The model under review builds one solid part; all positions refer to its coordinate system, in mm. A direction names the side the tool comes from. Coordinates: 2 decimals unless noted, no trailing zeros. Order: outer loops, then holes, each group sorted by start corner. A loop starts at its lowest first (then second) coordinate and runs counter-clockwise, first axis right, second up. Notation, with made-up numbers: (73.25, 49) -> (107.25, 49) arc R23 cw to (107.25, 83) -> close; hole circle Ø2 at (55.5, 88.25). An arc over 180 degrees is marked (long way). Use one line per item in the form item = value. Start each with the question number.
(1) Take a section at B-B (x = -4.5). State the section outline as (y, z) points, then the cut area to 3 significant figures.
(2) Take a section at A-A (y = -46). State the section outline as (x, z) points, then the cut area to 3 significant figures.
(3) Take a section at D-D (y = -24.5). State the section outline as (x, z) points.
(4) Insertion check: pin 1 Ø5.5 at (x, z) = (-18, 1.5) entering from -Y; pin 2 Ø1.5 at (x, y) = (-9.5, -18.5) entering from -Z; pin 3 Ø12 at (x, z) = (-1.5, 22) entering from +Y; pin 4 Ø21 at (x, y) = (-2.5, 5.5) entering from +Z. Each pin has a flat end and moves straight along its axis. Give the tip position at first contact, or say it passes through.
(5) For faces 5 (the flat face through (17, -35.5, 2)), 6 (the flat face through (-25.6, 27, 5)), 7 (the cylindrical face through (-6.232, -28.066, 6.479)), list the 3-axis set-ups (+Z, -Z, +X, -X, +Y, -Y) from which the entire face can be reached by the end or side of a thin tool; tool diameter is ignored.
(6) Take a section at C-C (z = 19.5). State the section outline as (x, y) points.
(7) Mouldability with a two-part tool opening along X and no side actions: class faces 1 (the cylindrical face through (29.038, 26.004, 2.465)), 2 (the cylindrical face through (33.245, -33.361, 2.465)), 3 (the flat face through (27, 25.7, 5)), 4 (the cylindrical face through (-33.361, -33.245, 2.465)) as +X half, -X half, draft (parallel to the pull), parting line (faces both ways), or undercut.
(8) Wall thickness on line 1 along Y through (x, z) = (28, 3.7); line 2 along Y through (x, z) = (0, 9.7); line 3 along Z through (x, y) = (-19.5, 16): over which ranges is each line inside the solid? List them lowest first.
```python
from build123d import *

# Parameters (mm, degrees)
SKETCH004_R         = 2.25
SKETCH004_R_2       = 11.1
SKETCH004_R_3       = 1.65
PAD005_DEPTH        = 5
SKETCH005_R         = 35.5
SKETCH005_R_2       = 32.6
PAD006_DEPTH        = 8
SKETCH070_R         = 32.6
SKETCH070_R_2       = 28.75
PAD045_DEPTH        = 3
SKETCH071_W         = 11
SKETCH071_H         = 18
SKETCH071_R         = 1.0922
PAD046_DEPTH        = 25.5
HOLE002_D           = 3.4
HOLE002_CSINK_D     = 6.7
HOLE002_CSINK_ANGLE = 90


with BuildPart() as part:
    # Sketch004 → Pad005 (new body)
    with BuildSketch(Plane.XY):
        with BuildLine():
            Line((-28, 35.5), (28, 35.5))
            ThreePointArc((35.5, 28), (33.303301, 33.303301), (28, 35.5))
            Line((35.5, 28), (35.5, -28))
            ThreePointArc((28, -35.5), (33.303301, -33.303301), (35.5, -28))
            Line((28, -35.5), (-28, -35.5))
            ThreePointArc((-35.5, -28), (-33.303301, -33.303301), (-28, -35.5))
            Line((-35.5, -28), (-35.5, 28))
            ThreePointArc((-28, 35.5), (-33.303301, 33.303301), (-35.5, 28))
        make_face()
        with Locations((-28, 28)):
            Circle(SKETCH004_R, mode=Mode.SUBTRACT)
        with Locations((28, 28)):
            Circle(SKETCH004_R, mode=Mode.SUBTRACT)
        with Locations((28, -28)):
            Circle(SKETCH004_R, mode=Mode.SUBTRACT)
        with Locations((-28, -28)):
            Circle(SKETCH004_R, mode=Mode.SUBTRACT)
        Circle(SKETCH004_R_2, mode=Mode.SUBTRACT)
        with Locations((-9.899495, 9.899495)):
            Circle(SKETCH004_R_3, mode=Mode.SUBTRACT)
        with Locations((9.899495, 9.899495)):
            Circle(SKETCH004_R_3, mode=Mode.SUBTRACT)
        with Locations((9.899495, -9.899495)):
            Circle(SKETCH004_R_3, mode=Mode.SUBTRACT)
        with Locations((-9.899495, -9.899495)):
            Circle(SKETCH004_R_3, mode=Mode.SUBTRACT)
    extrude(amount=PAD005_DEPTH)

    # Sketch005 → Pad006 (join)
    with BuildSketch(Plane.XY.offset(5)):
        Circle(SKETCH005_R)
        Circle(SKETCH005_R_2, mode=Mode.SUBTRACT)
    extrude(amount=PAD006_DEPTH)

    # Sketch070 → Pad045 (join)
    with BuildSketch(Plane.XY.offset(5)):
        Circle(SKETCH070_R)
        Circle(SKETCH070_R_2, mode=Mode.SUBTRACT)
    extrude(amount=PAD045_DEPTH)

    # Sketch071 → Pad046 (join)
    with BuildSketch(Plane.XY):
        with Locations((-0.5, -42)):
            Rectangle(SKETCH071_W, SKETCH071_H)
        with Locations((0, -38)):
            Circle(SKETCH071_R, mode=Mode.SUBTRACT)
        with Locations((0, -46)):
            Circle(SKETCH071_R, mode=Mode.SUBTRACT)
    extrude(amount=PAD046_DEPTH)

    # Hole002 (through all)
    with Locations(Plane.XY.offset(5)):
        with Locations((-9.899495, 9.899495), (9.899495, 9.899495), (9.899495, -9.899495), (-9.899495, -9.899495)):
            CounterSinkHole(HOLE002_D / 2, HOLE002_CSINK_D / 2, counter_sink_angle=HOLE002_CSINK_ANGLE)


solid = part.part
```
Findings:
q1.outline = (-51, 0) -> (-10.15, 0) -> (-10.15, 5) -> (-28.4, 5) -> (-28.4, 8) -> (-32.29, 8) -> (-32.29, 13) -> (-33, 13) -> (-33, 25.5) -> (-51, 25.5) -> close; (10.15, 0) -> (35.5, 0) -> (35.5, 5) -> (35.21, 5) -> (35.21, 13) -> (32.29, 13) -> (32.29, 8) -> (28.4, 8) -> (28.4, 5) -> (10.15, 5) -> close
q1.area = 752 mm²
q2.outline = (-6, 0) -> (-1.09, 0) -> (-1.09, 25.5) -> (-6, 25.5) -> close; (1.09, 0) -> (5, 0) -> (5, 25.5) -> (1.09, 25.5) -> close
q2.area = 225 mm²
q3.outline = (-35.5, 0) -> (35.5, 0) -> (35.5, 5) -> (25.69, 5) -> (25.69, 13) -> (21.51, 13) -> (21.51, 8) -> (15.04, 8) -> (15.04, 5) -> (-15.04, 5) -> (-15.04, 8) -> (-21.51, 8) -> (-21.51, 13) -> (-25.69, 13) -> (-25.69, 5) -> (-35.5, 5) -> close
q4.pin_1 = -35.5
q4.pin_2 = 0
q4.pin_3 = -33
q4.pin_4 = 5
q5.face_5 = +Z, -Z, +X, -Y
q5.face_6 = +Z, -X, +Y
q5.face_7 = +Z
q6.outline = (-6, -51) -> (5, -51) -> (5, -33) -> (-6, -33) -> close; hole circle Ø2.18 at (0, -46); hole circle Ø2.18 at (0, -38)
q7.face_1 = undercut
q7.face_2 = +X half
q7.face_3 = draft
q7.face_4 = -X half
q8.line_1 = -35.5 to -30.25, -25.75 to 25.75, 30.25 to 35.5
q8.line_2 = -51 to -47.09, -44.91 to -39.09, -36.91 to -32.6, 32.6 to 35.5
q8.line_3 = 0 to 5
